from build123d import *

# Parameters (mm, degrees)
SKETCH1_R           = 100
BOSS_EXTRUDE1_DEPTH = 5
SKETCH2_R           = 50
BOSS_EXTRUDE2_DEPTH = 5
SKETCH3_R           = 10
SKETCH3_R_2         = 5
BOSS_EXTRUDE3_DEPTH = 5
SKETCH5_R           = 22.5
BOSS_EXTRUDE4_DEPTH = 40
SKETCH6_R           = 55
BOSS_EXTRUDE5_DEPTH = 5
SKETCH7_R           = 15
BOSS_EXTRUDE6_DEPTH = 20
SKETCH9_R           = 2.5
CUT_EXTRUDE2_DEPTH  = 5
SKETCH11_R          = 10
CUT_EXTRUDE3_DEPTH  = 1


with BuildPart() as part:
    # Sketch1 → Boss-Extrude1 (new body)
    with BuildSketch(Plane(origin=(0, 0, 0), x_dir=(1, 0, 0), z_dir=(0, 1, 0))):
        with Locations(Location((0, 0, 0), (0, 0, 270))):
            Circle(SKETCH1_R)
    extrude(amount=BOSS_EXTRUDE1_DEPTH)



with BuildPart() as body_2:
    # Sketch2 → Boss-Extrude2 (new body)
    with BuildSketch(Plane(origin=(0, 15, 0), x_dir=(-1, 0, 0), z_dir=(0, -1, 0))):
        with Locations(Location((0, 0, 0), (0, 0, 90))):
            Circle(SKETCH2_R)
    extrude(amount=BOSS_EXTRUDE2_DEPTH)


with BuildPart() as part_1:
    add(part.part)

    add(body_2.part)  # Boss-Extrude3 merges body 2
    # Sketch3 → Boss-Extrude3 (add)
    with BuildSketch(Plane(origin=(0, 5, 0), x_dir=(1, 0, 0), z_dir=(0, 1, 0))):
        with Locations(Location((0, 0, 0), (0, 0, 90))):
            Circle(SKETCH3_R)
        with Locations(Location((0, 0, 0), (0, 0, 90))):
            Circle(SKETCH3_R_2, mode=Mode.SUBTRACT)
    extrude(amount=BOSS_EXTRUDE3_DEPTH)

    # Sketch4 → Revolve1 (revolve)
    with BuildSketch(Plane.XY, mode=Mode.PRIVATE) as revolve1_sk:
        Polygon((50, 15), (100, 5), (0, 5), (0, 10), (50, 10), align=None)
    revolve(revolve1_sk.sketch.rotate(Axis((0, 54.07219912, 0), (0, -1, 0)), 270), axis=Axis((0, 54.07219912, 0), (0, -1, 0)))

    # Sketch5 → Boss-Extrude4 (add)
    with BuildSketch(Plane.XZ):
        with Locations(Location((0, 0, 0), (0, 0, 270))):
            Circle(SKETCH5_R)
    extrude(amount=BOSS_EXTRUDE4_DEPTH)

    # Sketch6 → Boss-Extrude5 (add)
    with BuildSketch(Plane.XZ.offset(40)):
        with Locations(Location((0, 0, 0), (0, 0, 270))):
            Circle(SKETCH6_R)
    extrude(amount=BOSS_EXTRUDE5_DEPTH)

    # Sketch7 → Boss-Extrude6 (add)
    with BuildSketch(Plane.XZ.offset(45)):
        with Locations(Location((-25, -25, 0), (0, 0, 270))):
            Circle(SKETCH7_R)
        with Locations(Location((25, -25, 0), (0, 0, 270))):
            Circle(SKETCH7_R)
        with Locations(Location((25, 25, 0), (0, 0, 270))):
            Circle(SKETCH7_R)
        with Locations(Location((-25, 25, 0), (0, 0, 270))):
            Circle(SKETCH7_R)
    extrude(amount=BOSS_EXTRUDE6_DEPTH)

    # Sketch9 → Cut-Extrude2 (cut)
    with BuildSketch(Plane.XZ.offset(45)):
        with Locations(Location((0, 40, 0), (0, 0, 270))):
            Circle(SKETCH9_R)
        with Locations(Location((40, 0, 0), (0, 0, 270))):
            Circle(SKETCH9_R)
        with Locations(Location((0, -40, 0), (0, 0, 270))):
            Circle(SKETCH9_R)
        with Locations(Location((-40, 0, 0), (0, 0, 270))):
            Circle(SKETCH9_R)
    extrude(amount=-CUT_EXTRUDE2_DEPTH, mode=Mode.SUBTRACT)

    # Sketch11 → Cut-Extrude3 (cut)
    with BuildSketch(Plane(origin=(0, -40, 0), x_dir=(1, 0, 0), z_dir=(0, 1, 0))):
        with Locations(Location((0, 40, 0), (0, 0, 270))):
            Circle(SKETCH11_R)
        with Locations(Location((40, 0, 0), (0, 0, 270))):
            Circle(SKETCH11_R)
        with Locations(Location((0, -40, 0), (0, 0, 270))):
            Circle(SKETCH11_R)
        with Locations(Location((-40, 0, 0), (0, 0, 270))):
            Circle(SKETCH11_R)
    extrude(amount=-CUT_EXTRUDE3_DEPTH, mode=Mode.SUBTRACT)


solid = part_1.part
Check sheet for the modelled part. Datum: model origin and axes. Units: mm. A direction names the side the tool comes from. Coordinates: 2 decimals unless noted, no trailing zeros. Write each loop counter-clockwise with the first axis right and the second up, starting at its lowest first coordinate (ties: lowest second). Pieces come first, ordered by that corner, then holes. Notation, with made-up numbers: M 68.25,-36.75 L 85.25,-36.75 A27 cw 85.25,-8.75 Z; hole C 33.5,11.5 d10. An arc over 180 degrees is marked long. Answer as CSV lines item,"result".
Q1. Cross-section at A-A (z = 0). Count the separate pieces of the cut face and the enclosed holes in it, then the cut area to 3 significant figures.
Check result:
separate pieces,"3"
enclosed holes,"0"
area,"4,770 mm^2"
Q2. Material ranges on probe 1 along Y at (x, z) = (45, -10.5); probe 2 along Y at (x, z) = (11.5, 3.5); probe 3 along Y at (x, z) = (38, 19), recorded low to high. Write a range as from..to.
Check result:
probe 1,"-45..-40, 0..15"
probe 2,"-45..15"
probe 3,"-65..-40, 0..15"
Q3. Mould release check, pull along X, two halves, no side actions. Record for faces 4 (the face through (1, 15, 1)), 5 (the face through (-8.618, -19.72, -20.784)), 6 (the face through (37.56, -43.03, 0.54)): released by +X, released by -X, zero draft, split by the parting line, or undercut.
Check result:
face 4,"zero draft"
face 5,"split by the parting line"
face 6,"undercut"
Q4. Go/stop test with flat-tipped pins: pin 1 (1.5 mm diameter, centred on x = -56.5, z = 42, fed in from -Y); pin 2 (4 mm diameter, centred on x = 43.5, z = 52, fed in from +Y); pin 3 (6.5 mm diameter, centred on x = -40, z = 0, fed in from -Y). Record where each tip stops, or that it passes through.
Check result:
pin 1,"y = 0"
pin 2,"y = 11.84"
pin 3,"y = -45"
Q5. Cross-section at B-B (y = -34). Record the boundary of the cut face in (x, z).
Check result:
outline,"C 0,0 d45"
Q6. Set-up check for faces 1 (the face through (-2, -41, -38)), 2 (the face through (-25, -65, -25)), 3 (the face through (-39.643, -54.86, 28.252)): record each of +Z, -Z, +X, -X, +Y, -Y from which the full face is reachable in a straight line by a thin tool's end or side.
Check result:
face 1,"none"
face 2,"+Z, -Z, +X, -X, -Y"
face 3,"-Y"
